```python
from build123d import *

# Parameters (mm, degrees)
BOSS_EXTRU_1_DEPTH      = 25
ESQUISSE2_R             = 2.65
ENL_V_MAT_EXTRU_1_DEPTH = 28.166155414
ESQUISSE3_R             = 3.2
ENL_V_MAT_EXTRU_2_DEPTH = 1.5


with BuildPart() as part:
    # Esquisse1 → Boss.-Extru.1 (new body)
    with BuildSketch(Plane.XY):
        Polygon((0, 0), (7, 0), (7, 8), (0, 5), align=None)
    extrude(amount=BOSS_EXTRU_1_DEPTH)

    # Esquisse2 → Enlèv. mat.-Extru.1 (cut, through all)
    with BuildSketch(Plane.ZY):
        with Locations(Location((5, 4, 0), (0, 0, 270))):
            Circle(ESQUISSE2_R)
        with Locations(Location((12.5, 4, 0), (0, 0, 270))):
            Circle(ESQUISSE2_R)
        with Locations(Location((20, 4, 0), (0, 0, 270))):
            Circle(ESQUISSE2_R)
    extrude(amount=-ENL_V_MAT_EXTRU_1_DEPTH, mode=Mode.SUBTRACT)

    # Esquisse3 → Enlèv. mat.-Extru.2 (cut)
    with BuildSketch(Plane(origin=(7, 0, 0), x_dir=(0, 0, -1), z_dir=(1, 0, 0))):
        with Locations((-20, 4)):
            Circle(ESQUISSE3_R)
        with Locations((-12.5, 4)):
            Circle(ESQUISSE3_R)
        with Locations((-5, 4)):
            Circle(ESQUISSE3_R)
    extrude(amount=-ENL_V_MAT_EXTRU_2_DEPTH, mode=Mode.SUBTRACT)


solid = part.part
```
Work out the finished part from the listing and answer in its coordinate system (mm). A direction names the side the tool comes from. Give positions to 0.01 mm unless a question says otherwise; leave off trailing zeros. Loops run counter-clockwise (first coordinate to the right, second up) from the corner with the lowest first, then second, coordinate; pieces in that order, holes last. Notation, with made-up numbers: (89, 75) - (104, 75) arc R14 cw to (104, 95) - close; hole circle Ø7 at (75.25, 27). An arc over 180 degrees is marked (long way). One line per question, with ' | ' between items.
(1) The mould has two halves that part along Y. Classify faces 1 (the face through (3, 0, 12)), 2 (the face through (5.5, 7, 12)), 3 (the face through (4.327, 6.854, 12.325)), 4 (the face through (0, 1, 12)): +Y half, -Y half, draft (parallel to the pull), parting line (faces both ways), or undercut.
Recorded:
face 1: -Y half | face 2: undercut | face 3: +Y half | face 4: draft
(2) The part is cut by section A-A (z = 12.5). Write down the section's boundary in (x, y).
Recorded:
outline: (0, 0) - (7, 0) - (7, 0.8) - (5.5, 0.8) - (5.5, 1.35) - (0, 1.35) - close; (3.85, 6.65) - (5.5, 6.65) - (5.5, 7.2) - (7, 7.2) - (7, 8) - close
(3) A tool of negligible diameter and unlimited length cuts with its end or side. For faces 5 (the face through (6.3, 4.1, 23.2)), 6 (the face through (2.71, 1.55, 11.49)), from which of +Z, -Z, +X, -X, +Y, -Y can it reach the whole face along a straight path? Write none if from no direction.
Recorded:
face 5: +X | face 6: +X, -X
(4) Straight lines are drawn through the part: probe 1 along Z at (x, y) = (3, 4); probe 2 along Z at (x, y) = (3.75, 5.75); probe 3 along Y at (x, z) = (2.9, 12.5). For each, find the intervals that lie inside material, in ascending order.
Recorded:
probe 1: z = 0 to 2.35, 7.65 to 9.85, 15.15 to 17.35, 22.65 to 25 | probe 2: z = 0 to 3.01, 6.99 to 10.51, 14.49 to 18.01, 21.99 to 25 | probe 3: y = 0 to 1.35
(5) Each of these flat-tipped pins is pushed along its axis until it touches: pin 1 Ø2 at (x, z) = (4, 5) entering from +Y; pin 2 Ø3 at (x, z) = (1, 16.5) entering from +Y; pin 3 Ø3 at (x, z) = (0.5, 21.5) entering from +Y. Where does it stop, or does it pass through?
Recorded:
pin 1: stops at y = 7.14 | pin 2: stops at y = 6.07 | pin 3: stops at y = 5.83
(6) The part is cut by section D-D (y = 5.25). Write down the section's boundary in (x, z), then the cut area to 3 significant figures.
Recorded:
outline: (0.58, 0) - (7, 0) - (7, 2.05) - (5.5, 2.05) - (5.5, 2.66) - (0.58, 2.66) - close; (0.58, 7.34) - (5.5, 7.34) - (5.5, 7.95) - (7, 7.95) - (7, 9.55) - (5.5, 9.55) - (5.5, 10.16) - (0.58, 10.16) - close; (0.58, 14.84) - (5.5, 14.84) - (5.5, 15.45) - (7, 15.45) - (7, 17.05) - (5.5, 17.05) - (5.5, 17.66) - (0.58, 17.66) - close; (0.58, 22.34) - (5.5, 22.34) - (5.5, 22.95) - (7, 22.95) - (7, 25) - (0.58, 25) - close | area: 65.0 mm²
(7) The part is cut by section B-B (y = 4). Write down the section's boundary in (x, z).
Recorded:
outline: (0, 0) - (7, 0) - (7, 1.8) - (5.5, 1.8) - (5.5, 2.35) - (0, 2.35) - close; (0, 7.65) - (5.5, 7.65) - (5.5, 8.2) - (7, 8.2) - (7, 9.3) - (5.5, 9.3) - (5.5, 9.85) - (0, 9.85) - close; (0, 15.15) - (5.5, 15.15) - (5.5, 15.7) - (7, 15.7) - (7, 16.8) - (5.5, 16.8) - (5.5, 17.35) - (0, 17.35) - close; (0, 22.65) - (5.5, 22.65) - (5.5, 23.2) - (7, 23.2) - (7, 25) - (0, 25) - close
(8) The part is cut by section C-C (x = 6.75). Write down the section's boundary in (y, z), then the cut area to 3 significant figures.
Recorded:
outline: (0, 0) - (7.89, 0) - (7.89, 25) - (0, 25) - close; hole circle Ø6.4 at (4, 5); hole circle Ø6.4 at (4, 12.5); hole circle Ø6.4 at (4, 20) | area: 101 mm²
